For this review, use the dimensioned drawing (mm, ordinates from the lowest corner) and the shaded views. Coordinates: 2 decimals unless noted, no trailing zeros. Write each loop counter-clockwise with the first axis right and the second up, starting at its lowest first coordinate (ties: lowest second). Pieces come first, ordered by that corner, then holes. Notation, with made-up numbers: (48.25, 12.25) -> (99.25, 12.25) arc R7 cw to (99.25, 17.25) -> close; hole circle Ø7 at (8, 68). An arc over 180 degrees is marked (long way). Put each result on its own line as item: value. Start each with the question number.
Item 1: Consider section D-D on y = 7. Give the boundary of the cut face in (x, z).
Item 2: Consider section A-A on z = 0.7. Give the boundary of the cut face in (x, y).
Item 3: Consider section C-C on x = 10. Give the boundary of the cut face in (y, z), and give its area (3 significant figures).
Item 4: To check wall thickness, follow L1, parallel to Y at x = 119.5, z = 2; L2, parallel to X at y = 14.5, z = 1.4; L3, parallel to Y at x = 68.5, z = 0.65. State the ranges of each line that lie inside material, in increasing order.
Item 5: Consider section B-B on y = 34. Give the boundary of the cut face in (x, z), and give its area (3 significant figures).
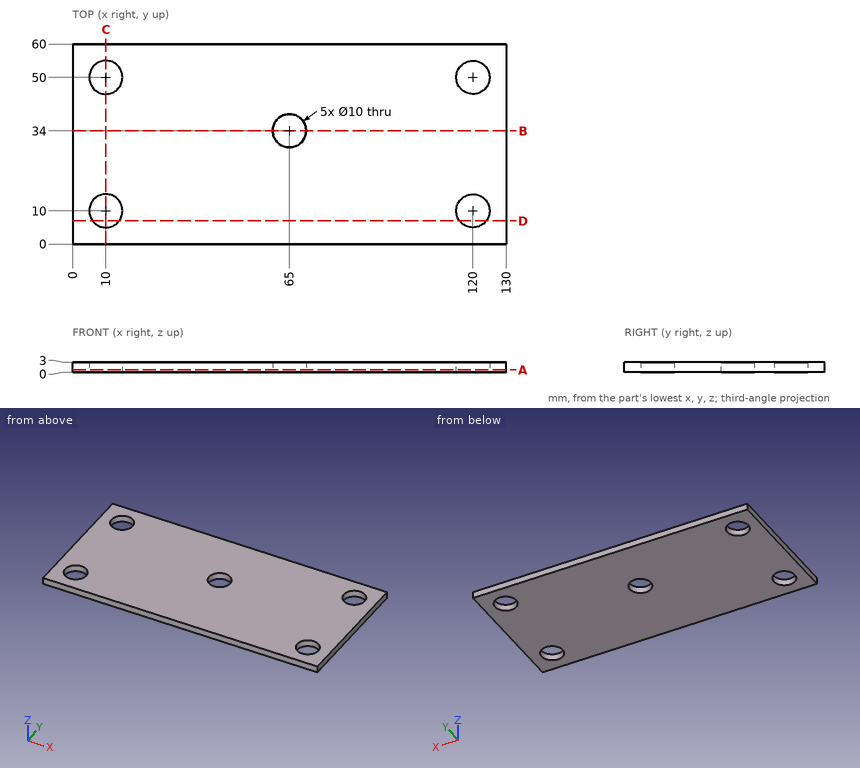
Return value:
1. outline: (0, 0) -> (6, 0) -> (6, 3) -> (0, 3) -> close; (14, 0) -> (116, 0) -> (116, 3) -> (14, 3) -> close; (124, 0) -> (130, 0) -> (130, 3) -> (124, 3) -> close
2. outline: (0, 0) -> (130, 0) -> (130, 60) -> (0, 60) -> close; hole circle Ø10 at (10, 10); hole circle Ø10 at (10, 50); hole circle Ø10 at (65, 34); hole circle Ø10 at (120, 10); hole circle Ø10 at (120, 50)
3. outline: (0, 0) -> (5, 0) -> (5, 3) -> (0, 3) -> close; (15, 0) -> (45, 0) -> (45, 3) -> (15, 3) -> close; (55, 0) -> (60, 0) -> (60, 3) -> (55, 3) -> close
3. area: 120 mm^2
4. L1: 0 to 5.03, 14.97 to 45.03, 54.97 to 60
4. L2: 0 to 7.82, 12.18 to 117.82, 122.18 to 130
4. L3: 0 to 30.43, 37.57 to 60
5. outline: (0, 0) -> (60, 0) -> (60, 3) -> (0, 3) -> close; (70, 0) -> (130, 0) -> (130, 3) -> (70, 3) -> close
5. area: 360 mm^2
